Verification items for the finished model (mm, model axes). Face numbers are marked on the shaded views. A direction names the side the tool comes from. Coordinates: 2 decimals unless noted, no trailing zeros. Write each loop counter-clockwise with the first axis right and the second up, starting at its lowest first coordinate (ties: lowest second). Pieces come first, ordered by that corner, then holes. Notation, with made-up numbers: (19, 13) -> (54, 13) arc R15 cw to (54, 28) -> close; hole circle Ø3 at (57, 82.5). An arc over 180 degrees is marked (long way). Write item = value, one per line. Start each with the question number.
(1) Set-up check for the marked faces 1, 2, 3 and 4: record each of +Z, -Z, +X, -X, +Y, -Y from which the full face is reachable in a straight line by a thin tool's end or side.
(2) Section check B-B (z = 6). Record the cut outline in (x, y) (3 decimals).
(3) Section check A-A (x = -69). Record the cut outline in (y, z) (3 decimals), plus the area to 3 significant figures.
(4) Mould release check, pull along X, two halves, no side actions. Record for the marked faces 5, 6, 7 and 8: released by +X, released by -X, zero draft, split by the parting line, or undercut.
(5) Gauge pin test, flat ends, axial feed: pin 1 Ø3.5 at (x, z) = (-69.5, 5) entering from +Y; pin 2 Ø1.3 at (y, z) = (1.5, 6.5) entering from -X; pin 3 Ø3.5 at (y, z) = (2.5, 4.5) entering from +X. Record the tip position at first contact, or that the pin passes through.
(6) Material ranges on probe 1 along Z at (x, y) = (-69.75, 4); probe 2 along Y at (x, z) = (-66.5, 5.25) (3 decimals); probe 3 along X at (y, z) = (0.5, 5.75), recorded low to high. Write a range as [from, to].
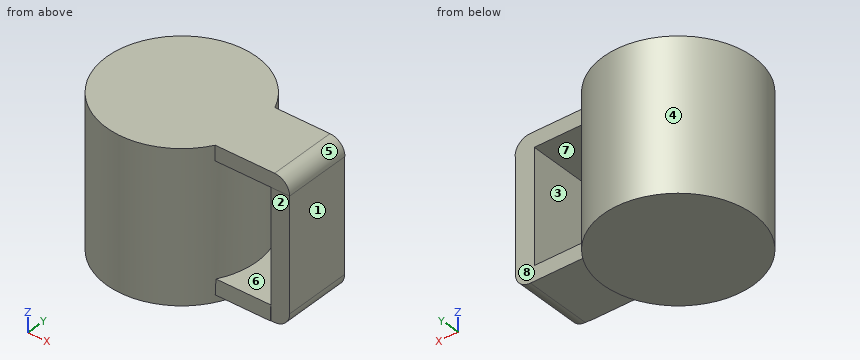
```python
from build123d import *

# Parameters (mm, degrees)
SKETCH_1_R      = 5
EXTRUDE_1_DEPTH = 10
SKETCH_9_W      = 7.120641766
SKETCH_9_H      = 4.534999238
EXTRUDE_6_DEPTH = 1
SKETCH_11_W     = 1.257653538
SKETCH_11_H     = 9
EXTRUDE_7_DEPTH = 4.5
EXTRUDE_8_DEPTH = 6
FILLET_8_R      = 1
FILLET_9_R      = 1


with BuildPart() as part:
    # Sketch 1 → Extrude 1 (new body)
    with BuildSketch(Plane(origin=(0.382706605, 0, 0), x_dir=(1, 0, 0), z_dir=(0, 0, 1))):
        with Locations((-75.594417438, 2.55)):
            Circle(SKETCH_1_R)
    extrude(amount=EXTRUDE_1_DEPTH)

    # Sketch 9 → Extrude 6 (add)
    with BuildSketch(Plane(origin=(6.127831546, 0, 9), x_dir=(1, 0, 0), z_dir=(0, 0, 1))):
        with Locations((-75.644850643, 2.267499619)):
            Rectangle(SKETCH_9_W, SKETCH_9_H)
    extrude(amount=EXTRUDE_6_DEPTH)



with BuildPart() as body_2:
    # Sketch 11 → Extrude 7 (new body)
    with BuildSketch(Plane(origin=(9.574526933, 4.534999238, 0.48426017), x_dir=(1, 0, 0), z_dir=(0, 1, 0))):
        with Locations((-76.184774061, -4.5)):
            Rectangle(SKETCH_11_W, SKETCH_11_H)
    extrude(amount=-EXTRUDE_7_DEPTH)


with BuildPart() as part_1:
    add(part.part)

    add(body_2.part)  # Extrude 8 merges body 2
    # Sketch 12 → Extrude 8 (add)
    with BuildSketch(Plane.ZY.offset(67.239073897)):
        Polygon((0.48426017, 4.534999238), (0.48426017, 0), (1.483647509, 0.034999238), (1.483647509, 4.534999238), align=None)
    extrude(amount=EXTRUDE_8_DEPTH)

    # Fillet 8
    fillet_8_edges = [part_1.edges().sort_by_distance(p)[0] for p in [
        (-65.981420359, 2.284999238, 0.48426017),
    ]]
    fillet(fillet_8_edges, radius=FILLET_8_R)

    # Fillet 9
    fillet_9_edges = [part_1.edges().sort_by_distance(p)[0] for p in [
        (-65.956698214, 2.267499619, 10),
    ]]
    fillet(fillet_9_edges, radius=FILLET_9_R - 0.0001)  # a hair under: the kernel refuses the full size


solid = part_1.part
```
Response:
q1.face_1 = -Z, +X, +Y, -Y
q1.face_2 = -Z, +X, -Y
q1.face_3 = +Y, -Y
q1.face_4 = none
q2.outline = circle Ø10 at (-75.212, 2.55); (-67.239, 0.035) -> (-65.981, 0.035) -> (-65.981, 4.535) -> (-67.239, 4.535) -> close
q3.outline = (0, 0.484) -> (4.535, 0.484) -> (4.535, 1.484) -> (0.035, 1.484) -> close; (0, 9) -> (4.535, 9) -> (4.535, 10) -> (0, 10) -> close
q3.area = 9.05 mm2
q4.face_5 = released by +X
q4.face_6 = undercut
q4.face_7 = undercut
q4.face_8 = zero draft
q5.pin_1 = 5.6
q5.pin_2 = -80.2
q5.pin_3 = -65.98
q6.probe_1 = [0.48, 1.48], [9, 10]
q6.probe_2 = [0.035, 4.535]
q6.probe_3 = [-79.77, -70.65], [-67.24, -65.98]
